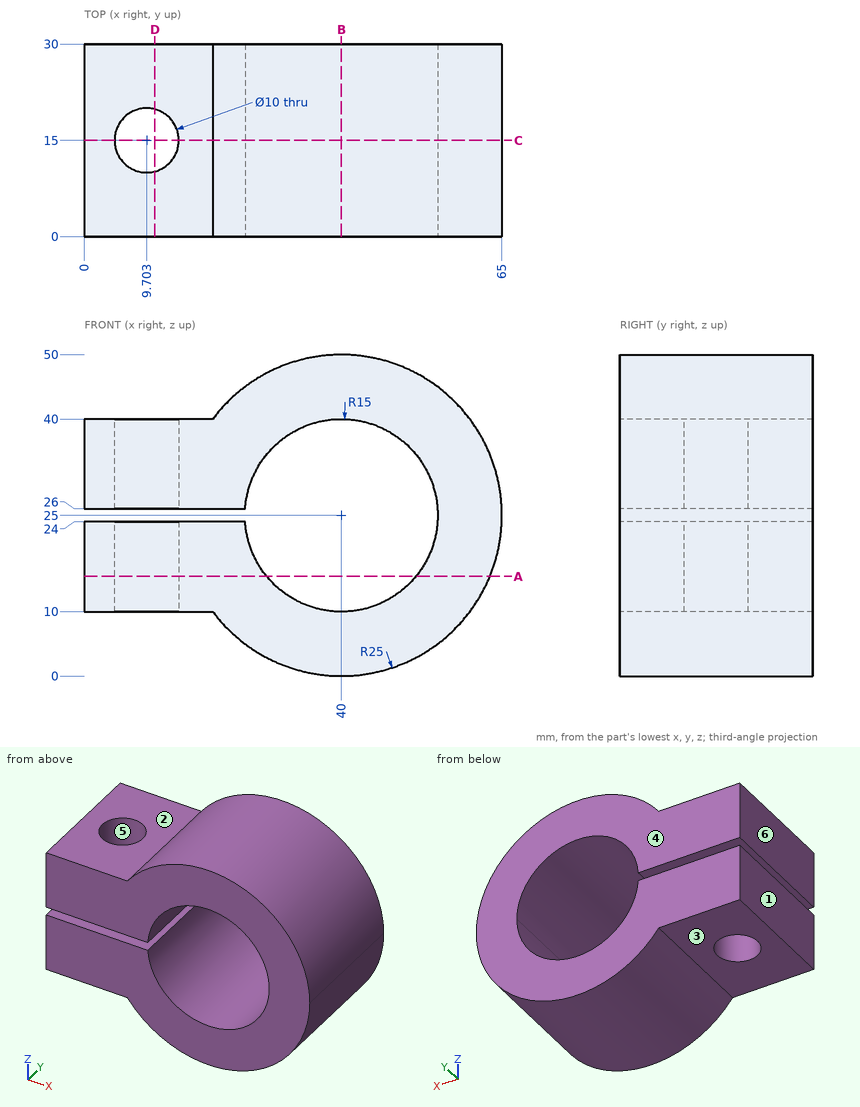
Geometry: see drawing. Coordinates: mm, zero at the bounding-box minimum. A direction names the side the tool comes from. Round coordinates to 2 decimals unless told otherwise and drop trailing zeros. Loops run counter-clockwise (first coordinate to the right, second up) from the corner with the lowest first, then second, coordinate; pieces in that order, holes last. Notation, with made-up numbers: (19, 15) - (50, 15) arc R9 ccw to (50, 19) - close; hole circle Ø10 at (85.5, -13.5). An arc over 180 degrees is marked (long way). Write item = value, one per line. Start each with the question number.
(1) Pull-direction query (Y, two-part tool) for the marked faces 4, 5 and 6; classes: +Y half, -Y half, draft (parallel to the pull), parting line (faces both ways), or undercut.
(2) Section query C-C, the plane y = 15. Output: boundary loops of the cut face in (x, z).
(3) Ray query, line 1 along X through (y, z) = (12.5, 30.5) (1 decimal); line 2 along X through (y, z) = (16.5, 37.5); line 3 along Z through (x, y) = (35, 5) (3 decimals). Return the intervals inside material, ascending. Write a range as from..to.
(4) Section query B-B, the plane x = 40. Output: boundary loops of the cut face in (y, z).
(5) Section query A-A, the plane z = 15.5. Output: boundary loops of the cut face in (x, y).
(6) Pin query (flat end, axial travel): pin 1 (1.5 mm diameter, centred on y = 8.5, z = 33.5, fed in from -X); pin 2 (7.5 mm diameter, centred on x = 7, y = 10.5, fed in from -Z); pin 3 (1 mm diameter, centred on x = 43.5, y = 5, fed in from +Z); pin 4 (8 mm diameter, centred on y = 10.5, z = 20, fed in from +X). Return the tip coordinate at first contact, or that it passes through.
(7) Set-up query: the marked faces 1, 2 and 3. Return all of +Z, -Z, +X, -X, +Y, -Y with unobstructed straight access to the full face (end or side cutting, diameter ignored); none if empty.
(8) Section query D-D, the plane x = 11. Output: boundary loops of the cut face in (y, z).
Conclusion:
q1.face_4 = +Y half
q1.face_5 = undercut
q1.face_6 = draft
q2.outline = (0, 10) - (4.7, 10) - (4.7, 24) - (0, 24) - close; (0, 26) - (4.7, 26) - (4.7, 40) - (0, 40) - close; (14.7, 10) - (20, 10) arc R25 ccw (long way) to (20, 40) - (14.7, 40) - (14.7, 26) - (25.03, 26) arc R15 cw (long way) to (25.03, 24) - (14.7, 24) - close
q3.line_1 = 0..5.4, 14..26, 54..64.4
q3.line_2 = 0..4.93, 14.47..31.71, 48.29..61.65
q3.line_3 = 0.505..10.858, 39.142..49.495
q4.outline = (0, 0) - (30, 0) - (30, 10) - (0, 10) - close; (0, 40) - (30, 40) - (30, 50) - (0, 50) - close
q5.outline = (0, 0) - (28.39, 0) - (28.39, 30) - (0, 30) - close; (51.61, 0) - (63.12, 0) - (63.12, 30) - (51.61, 30) - close; hole circle Ø10 at (9.7, 15)
q6.pin_1 = 0
q6.pin_2 = 10
q6.pin_3 = 49.82
q6.pin_4 = 64.98
q7.face_1 = +Z, -Z, -X, +Y, -Y
q7.face_2 = +Z, -X, +Y, -Y
q7.face_3 = -Z, -X, +Y, -Y
q8.outline = (0, 10) - (10.17, 10) - (10.17, 24) - (0, 24) - close; (0, 26) - (10.17, 26) - (10.17, 40) - (0, 40) - close; (19.83, 10) - (30, 10) - (30, 24) - (19.83, 24) - close; (19.83, 26) - (30, 26) - (30, 40) - (19.83, 40) - close
